```python
from build123d import *

# Parameters (mm, degrees)
SKETCH1_W          = 3
SKETCH1_H          = 157
SKETCH3_R          = 2
CUT_EXTRUDE1_DEPTH = 158.097591383


with BuildPart() as part:
    # Sketch1 → Revolve1 (revolve)
    with BuildSketch(Plane.XY.offset(1.653301878)):
        with Locations((1.5, -78.5)):
            Rectangle(SKETCH1_W, SKETCH1_H)
    revolve(axis=Axis((0, 0, 1.653301878), (0, -1, 0)))

    # Sketch3 → Cut-Extrude1 (cut, through all)
    with BuildSketch(Plane(origin=(0, 0, 0), x_dir=(1, 0, 0), z_dir=(0, 1, 0))):
        with Locations(Location((0, -1.653301878, 0), (0, 0, 180))):
            Circle(SKETCH3_R)
    extrude(amount=-CUT_EXTRUDE1_DEPTH, mode=Mode.SUBTRACT)


with BuildPart() as part_1:
    # Body-Move/Copy1: read off the stored shape, not the designer's step
    # Body-Move/Copy1: moved
    add(part.part.moved(Location((0, 157, -1.6533019))))


solid = part_1.part
```
Could you check a few things on this model? Use its own coordinates, in mm. Round coordinates to 2 decimals unless told otherwise and drop trailing zeros. Loops run counter-clockwise (first coordinate to the right, second up) from the corner with the lowest first, then second, coordinate; pieces in that order, holes last.
Q1. I want a section at B-B (x = 0). Write out the boundary of the cut face in (y, z).
Q2. I want a section at C-C (y = 89). Write out the boundary of the cut face in (x, z), and give its area (3 significant figures).
Q3. I want a section at A-A (z = 0). Write out the boundary of the cut face in (x, y).
Q4. Thinking about a two-plate mould opening in X: for faces 1 (the cylindrical face through (-3, 80, 0)), 2 (the flat face through (-1, 0, -2)), 3 (the cylindrical face through (0, 80, 2)), which applies, pulls with the +X half, pulls with the -X half, needs draft (parallel to the pull), parting line crosses it, or undercut?
Q5. Please list where these lines run through material, in increasing order: L1, parallel to Z at x = 0, y = 73.5; L2, parallel to X at y = 144, z = 0.15; L3, parallel to X at y = 68, z = 0.8.
Q6. For P1, Ø1, axis at y = 111, z = -1.5, coming from the +X side; P2, Ø1.5, axis at y = 102, z = -1, coming from the -X side, each with a flat end and sliding along its axis, tell me the tip position at first contact or that it passes through.
Answer below:
1. outline: (0, -3) - (157, -3) - (157, -2) - (0, -2) - close; (0, 2) - (157, 2) - (157, 3) - (0, 3) - close
2. outline: circle Ø6 at (0, 0); hole circle Ø4 at (0, 0)
2. area: 15.7 mm2
3. outline: (-3, 0) - (-2, 0) - (-2, 157) - (-3, 157) - close; (2, 0) - (3, 0) - (3, 157) - (2, 157) - close
4. face 1: parting line crosses it
4. face 2: needs draft
4. face 3: undercut
5. L1: z = -3 to -2, 2 to 3
5. L2: x = -3 to -1.99, 1.99 to 3
5. L3: x = -2.89 to -1.83, 1.83 to 2.89
6. P1: stops at x = 2.83
6. P2: stops at x = -2.99
